Could you check a few things on this model? Use its own coordinates, in mm. Face numbers are marked on the shaded views. A direction names the side the tool comes from. Give positions to 0.01 mm unless a question says otherwise; leave off trailing zeros. Write each loop counter-clockwise with the first axis right and the second up, starting at its lowest first coordinate (ties: lowest second). Pieces come first, ordered by that corner, then holes. Notation, with made-up numbers: (38, -17.75) - (56, -17.75) arc R20 cw to (56, 0.25) - close; hole circle Ø6 at (35.25, -26). An arc over 180 degrees is marked (long way). Answer as CSV lines item,"result". Start each with the question number.
Q1. Imagine slicing it at D-D on y = 35. List the corners of the cut face in (x, z) for me, and give its area (3 significant figures).
Q2. If I drill on line 1 along Y through (x, z) = (-55.5, 10.25); line 2 along X through (y, z) = (12, 10.75); line 3 along Y through (x, z) = (-53, 19.5), over which ranges is the centre line in solid material (lowest first)?
Q3. Imagine slicing it at A-A on x = 23. List the corners of the cut face in (y, z) for me, and give its area (3 significant figures).
Q4. Imagine slicing it at C-C on z = 4. List the corners of the cut face in (x, y) for me.
Q5. Will these pins go through, and if not, where does the flat tip stop? pin 1 Ø1.5 at (y, z) = (5, 10) entering from -X; pin 2 Ø5 at (x, z) = (46.5, 14.5) entering from +Y; pin 3 Ø6 at (y, z) = (52.5, 19.5) entering from +X.
Q6. We'd pull the mould along X, two halves only. Please class the marked faces 1, 2, 3 and 4: pulls with the +X half, pulls with the -X half, needs draft (parallel to the pull), parting line crosses it, or undercut.
Q7. On a 3-axis mill with a long thin cutter (end or side, diameter ignored), from which of +Z, -Z, +X, -X, +Y, -Y can I reach the whole of each face in a straight line? I mean the marked faces 5 and 6. Say none if no direction works.
Q8. Imagine slicing it at B-B on y = 13. List the corners of the cut face in (x, z) for me.
```python
from build123d import *

# Parameters (mm, degrees)
F0_R     = 10
F0_R_2   = 5
F1_DEPTH = 25


with BuildPart() as f1:
    # F0 (on Top) → F1 (new body)
    with BuildSketch(Plane.XY):
        with BuildLine():
            ThreePointArc((-80.264366, 10.813902), (-74.406502, -3.328234), (-60.264366, -9.186098))
            Line((-60.264366, -9.186098), (49.735634, -9.186098))
            ThreePointArc((49.735634, -9.186098), (56.806702, -6.257166), (59.735634, 0.813902))
            Line((59.735634, 0.813902), (59.735634, 10.813902))
            ThreePointArc((59.735634, 10.813902), (56.806702, 17.88497), (49.735634, 20.813902))
            Line((49.735634, 20.813902), (39.735634, 20.813902))
            ThreePointArc((39.735634, 20.813902), (32.664566, 23.742834), (29.735634, 30.813902))
            Line((29.735634, 30.813902), (29.735634, 40.813902))
            ThreePointArc((29.735634, 40.813902), (26.806702, 47.88497), (19.735634, 50.813902))
            Line((19.735634, 50.813902), (9.735634, 50.813902))
            ThreePointArc((9.735634, 50.813902), (2.664566, 53.742834), (-0.264366, 60.813902))
            Line((-0.264366, 60.813902), (-0.264366, 70.813902))
            ThreePointArc((-0.264366, 70.813902), (-3.193298, 77.88497), (-10.264366, 80.813902))
            Line((-10.264366, 80.813902), (-60.264366, 80.813902))
            ThreePointArc((-60.264366, 80.813902), (-74.406502, 74.956037), (-80.264366, 60.813902))
            Line((-80.264366, 60.813902), (-80.264366, 10.813902))
        make_face()
        with Locations((-60.264366, 10.813902)):
            Circle(F0_R, mode=Mode.SUBTRACT)
        with Locations((49.735634, 10.813902)):
            Circle(F0_R_2, mode=Mode.SUBTRACT)
        with Locations((-60.264366, 64.266279)):
            Circle(F0_R, mode=Mode.SUBTRACT)
        with Locations((-10.264366, 68.882748)):
            Circle(F0_R_2, mode=Mode.SUBTRACT)
        with Locations((19.735634, 37.721559)):
            Circle(F0_R_2, mode=Mode.SUBTRACT)
    extrude(amount=F1_DEPTH)


solid = f1.part
```
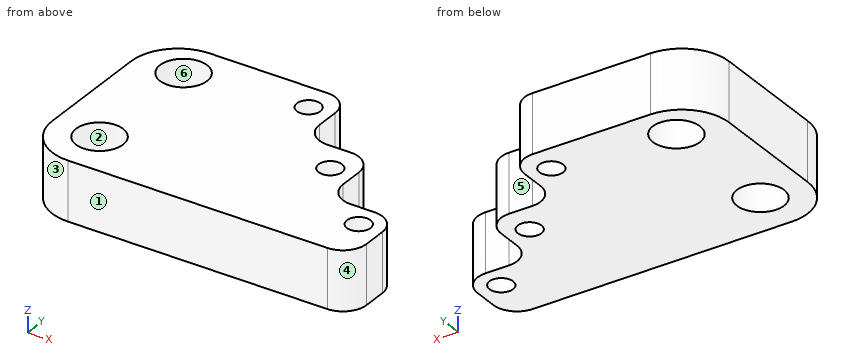
Conclusion:
1,outline,"(-80.26, 0) - (15.54, 0) - (15.54, 25) - (-80.26, 25) - close; (23.93, 0) - (29.74, 0) - (29.74, 25) - (23.93, 25) - close"
1,area,"2,540 mm^2"
2,line 1,"-9.19 to 2.02, 19.61 to 55.47, 73.06 to 80.81"
2,line 2,"-80.26 to -70.19, -50.33 to 44.88, 54.59 to 59.67"
2,line 3,"-9.19 to 3.94, 17.69 to 57.39, 71.14 to 80.81"
3,outline,"(-9.19, 0) - (33.93, 0) - (33.93, 25) - (-9.19, 25) - close; (41.51, 0) - (50.27, 0) - (50.27, 25) - (41.51, 25) - close"
3,area,"1,300 mm^2"
4,outline,"(-80.26, 10.81) arc R20 ccw to (-60.26, -9.19) - (49.74, -9.19) arc R10 ccw to (59.74, 0.81) - (59.74, 10.81) arc R10 ccw to (49.74, 20.81) - (39.74, 20.81) arc R10 cw to (29.74, 30.81) - (29.74, 40.81) arc R10 ccw to (19.74, 50.81) - (9.74, 50.81) arc R10 cw to (-0.26, 60.81) - (-0.26, 70.81) arc R10 ccw to (-10.26, 80.81) - (-60.26, 80.81) arc R20 ccw to (-80.26, 60.81) - close; hole circle Ø20 at (-60.26, 10.81); hole circle Ø20 at (-60.26, 64.27); hole circle Ø10 at (-10.26, 68.88); hole circle Ø10 at (19.74, 37.72); hole circle Ø10 at (49.74, 10.81)"
5,pin 1,"x = -79.61"
5,pin 2,"y = 20.81"
5,pin 3,"x = 24.69"
6,face 1,"needs draft"
6,face 2,"undercut"
6,face 3,"pulls with the -X half"
6,face 4,"pulls with the +X half"
7,face 5,"+Z, -Z, +X, +Y"
7,face 6,"+Z, -Z"
8,outline,"(-80.26, 0) - (-70.02, 0) - (-70.02, 25) - (-80.26, 25) - close; (-50.51, 0) - (45.24, 0) - (45.24, 25) - (-50.51, 25) - close; (54.23, 0) - (59.49, 0) - (59.49, 25) - (54.23, 25) - close"
